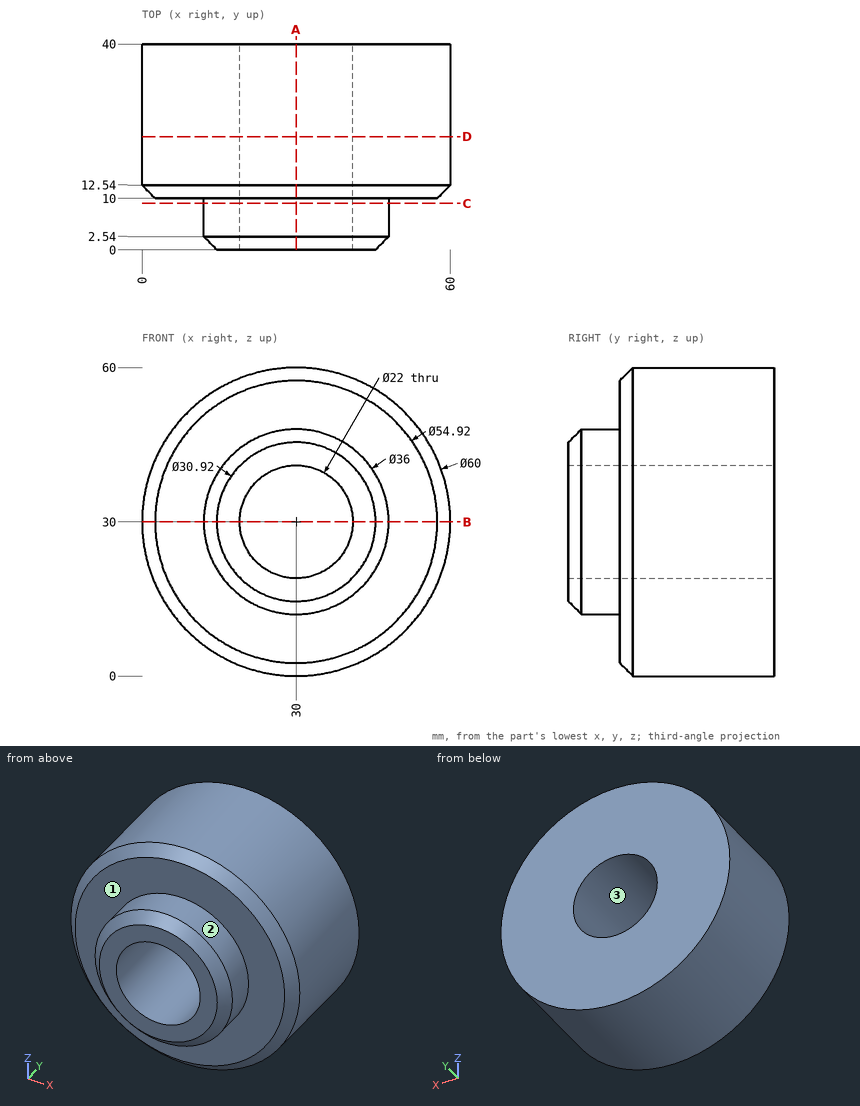
Answer from the drawing. Dimensions are ordinates in mm from the lowest x, y and z of the part. Round coordinates to 2 decimals unless told otherwise and drop trailing zeros. Write each loop counter-clockwise with the first axis right and the second up, starting at its lowest first coordinate (ties: lowest second). Pieces come first, ordered by that corner, then holes. Notation, with made-up numbers: M 32,73 L 37,73 A24 ccw 37,112 Z; hole C 22.5,0.25 d7. An arc over 180 degrees is marked long. Write each question's results on one line, items separated by ' | '. Start each with the question number.
Item 1: Given pin 1 Ø1 at (x, z) = (21.5, 27.5) entering from +Y; pin 2 Ø10 at (y, z) = (16, 22) entering from +X; pin 3 Ø5 at (x, y) = (24, 31.5) entering from +Z; pin 4 Ø4 at (y, z) = (13, 36.5) entering from -X, each flat-ended and moving along its own axis, determine where each tip first touches the part or whether it passes through.
Item 2: The mould has two halves that part along X. Classify the marked faces 1, 2 and 3: +X half, -X half, draft (parallel to the pull), parting line (faces both ways), or undercut.
Item 3: Find section D-D on y = 22. Write down the section's boundary in (x, z).
Item 4: Find section B-B on z = 30. Write down the section's boundary in (x, y), and give its area (3 significant figures).
Item 5: Find section C-C on y = 9. Write down the section's boundary in (x, z), and give its area (3 significant figures).
Item 6: Straight lines are drawn through the part: probe 1 along Z at (x, y) = (30, 23); probe 2 along Z at (x, y) = (30, 9); probe 3 along Y at (x, z) = (49.5, 17). For each, find the intervals that lie inside material, in ascending order.
Item 7: Find section A-A on x = 30. Write down the section's boundary in (y, z), and give its area (3 significant figures).
Answer block:
1) pin 1: passes through | pin 2: stops at x = 59.85 | pin 3: stops at z = 59.8 | pin 4: stops at x = 0.34
2) face 1: draft | face 2: parting line | face 3: undercut
3) outline: C 30,30 d60; hole C 30,30 d22
4) outline: M 0,12.54 L 2.54,10 L 12,10 L 12,2.54 L 14.54,0 L 19,0 L 19,40 L 0,40 Z; M 41,0 L 45.46,0 L 48,2.54 L 48,10 L 57.46,10 L 60,12.54 L 60,40 L 41,40 Z | area: 1,270 mm²
5) outline: C 30,30 d36; hole C 30,30 d22 | area: 638 mm²
6) probe 1: z = 0 to 19, 41 to 60 | probe 2: z = 12 to 19, 41 to 48 | probe 3: y = 10 to 40
7) outline: M 0,14.54 L 2.54,12 L 10,12 L 10,2.54 L 12.54,0 L 40,0 L 40,19 L 0,19 Z; M 0,41 L 40,41 L 40,60 L 12.54,60 L 10,57.46 L 10,48 L 2.54,48 L 0,45.46 Z | area: 1,270 mm²
